from build123d import *

# Parameters (mm, degrees)
F0_R     = 56.25
F0_R_2   = 1.225
F0_R_3   = 48.75
F1_DEPTH = 6
F2_R     = 1.5
F3_DEPTH = 5.9
F4_R     = 0.5


with BuildPart() as f1:
    # F0 (on Top) → F1 (new body)
    with BuildSketch(Plane.XY):
        Circle(F0_R)
        with Locations((-49.932854, -16.224168)):
            Circle(F0_R_2, mode=Mode.SUBTRACT)
        with Locations((0, -52.50251)):
            Circle(F0_R_2, mode=Mode.SUBTRACT)
        with Locations((49.932854, -16.224168)):
            Circle(F0_R_2, mode=Mode.SUBTRACT)
        with Locations((-30.860201, 42.475423)):
            Circle(F0_R_2, mode=Mode.SUBTRACT)
        Circle(F0_R_3, mode=Mode.SUBTRACT)
        with Locations((30.860201, 42.475423)):
            Circle(F0_R_2, mode=Mode.SUBTRACT)
    extrude(amount=F1_DEPTH)

    # F2
    f2_edges = [f1.edges().sort_by_distance(p)[0] for p in [
        (-48.75, 0, 6),
    ]]
    fillet(f2_edges, radius=F2_R)

    # F0 (on Top) → F3 (join)
    with BuildSketch(Plane.XY):
        Circle(F0_R)
        with Locations((-49.932854, -16.224168)):
            Circle(F0_R_2, mode=Mode.SUBTRACT)
        with Locations((0, -52.50251)):
            Circle(F0_R_2, mode=Mode.SUBTRACT)
        with Locations((49.932854, -16.224168)):
            Circle(F0_R_2, mode=Mode.SUBTRACT)
        with Locations((-30.860201, 42.475423)):
            Circle(F0_R_2, mode=Mode.SUBTRACT)
        Circle(F0_R_3, mode=Mode.SUBTRACT)
        with Locations((30.860201, 42.475423)):
            Circle(F0_R_2, mode=Mode.SUBTRACT)
    extrude(amount=F3_DEPTH)

    # F4
    f4_edges = [f1.edges().sort_by_distance(p)[0] for p in [
        (-48.75, 0, 0),
        (-56.25, 0, 0),
        (-56.25, 0, 6),
    ]]
    fillet(f4_edges, radius=F4_R)


solid = f1.part
Work out the finished part from the listing and answer in its coordinate system (mm). A direction names the side the tool comes from. Round coordinates to 2 decimals unless told otherwise and drop trailing zeros. Loops run counter-clockwise (first coordinate to the right, second up) from the corner with the lowest first, then second, coordinate; pieces in that order, holes last. Notation, with made-up numbers: (70, 88.25) - (84, 88.25) arc R16 cw to (84, 111.25) - close; hole circle Ø4 at (21.5, 34). An arc over 180 degrees is marked (long way). One line per item, written item: value.
Q1. The mould has two halves that part along Y. Classify faces 1 (the cylindrical face through (30.7, 43.69, 2.96)), 2 (the cylindrical face through (-56.196, 2.473, 2.965)), 3 (the flat face through (-50, 9, 6)): +Y half, -Y half, draft (parallel to the pull), parting line (faces both ways), or undercut.
Check values:
face 1: undercut
face 2: parting line
face 3: draft
Q2. Find section B-B on z = 1.5. Give the vertices of the cut face in (x, y) (3 decimals).
Check values:
outline: circle Ø112.5 at (0, 0); hole circle Ø2.45 at (-49.933, -16.224); hole circle Ø97.5 at (0, 0); hole circle Ø2.45 at (-30.86, 42.475); hole circle Ø2.45 at (0, -52.503); hole circle Ø2.45 at (30.86, 42.475); hole circle Ø2.45 at (49.933, -16.224)
Q3. Straight lines are drawn through the part: probe 1 along Y at (x, z) = (0, 2.6); probe 2 along Y at (x, z) = (-1.5, 5.5); probe 3 along X at (y, z) = (36, 4.7). For each, find the intervals that lie inside material, in ascending order.
Check values:
probe 1: -56.25 to -53.73, -51.28 to -48.75, 48.75 to 56.25
probe 2: -56.23 to -48.73, 48.73 to 56.23
probe 3: -43.22 to -32.87, 32.87 to 43.22
Q4. Find section A-A on y = 0. Give the vertices of the cut face in (x, z), and give its area (3 significant figures).
Check values:
outline: (-56.25, 0.5) arc R0.5 ccw to (-55.75, 0) - (-49.25, 0) arc R0.5 ccw to (-48.75, 0.5) - (-48.75, 5.9) - (-49.71, 5.9) arc R1.5 ccw to (-50.25, 6) - (-55.75, 6) arc R0.5 ccw to (-56.25, 5.5) - close; (48.75, 0.5) arc R0.5 ccw to (49.25, 0) - (55.75, 0) arc R0.5 ccw to (56.25, 0.5) - (56.25, 5.5) arc R0.5 ccw to (55.75, 6) - (50.25, 6) arc R1.5 ccw to (49.71, 5.9) - (48.75, 5.9) - close
area: 89.5 mm2
Q5. For faces 4 (the flat face through (49.3, -3.9, 0)), 5 (the flat face through (32.9, -36.6, 5.9)), determine the directions among +Z, -Z, +X, -X, +Y, -Y from which every point of the face is accessible in a straight line to the end or side of a thin tool.
Check values:
face 4: -Z, +X, -X, +Y, -Y
face 5: +Z
Q6. Each of these flat-tipped pins is pushed along its axis until it touches: pin 1 Ø3 at (x, z) = (25.5, 5) entering from +Y; pin 2 Ø3 at (x, y) = (-39.5, -27) entering from +Z; pin 3 Ø1 at (x, z) = (20.5, 1.5) entering from +Y. Where does it stop, or does it pass through?
Check values:
pin 1: y = 50.87
pin 2: z = 5.9
pin 3: y = 52.57
